Work out the finished part from the listing and answer in its coordinate system (mm). Round coordinates to 2 decimals unless told otherwise and drop trailing zeros. Write each loop counter-clockwise with the first axis right and the second up, starting at its lowest first coordinate (ties: lowest second). Pieces come first, ordered by that corner, then holes. Notation, with made-up numbers: (-39.5, 79.5) - (11.5, 79.5) arc R23 ccw to (11.5, 116.5) - close; hole circle Ø5 at (43.5, -20). An arc over 180 degrees is marked (long way). Answer as a JSON object with one key per item and string values.
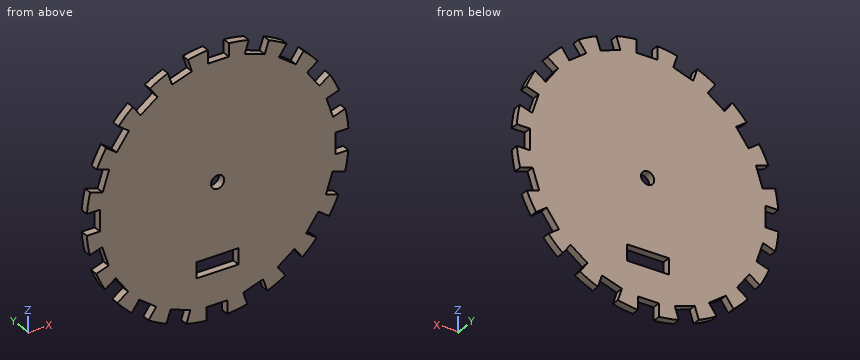
```python
from build123d import *

# Parameters (mm, degrees)
SKETCH1_R           = 50
BOSS_EXTRUDE3_DEPTH = 3
SKETCH7_R           = 2.5
CUT_EXTRUDE1_DEPTH  = 3
CUT_EXTRUDE4_START  = -3
CUT_EXTRUDE4_DEPTH  = 74.774289117
CIRPATTERN5_COUNT   = 20
SKETCH9_W           = 16
SKETCH9_H           = 6
CUT_EXTRUDE5_DEPTH  = 3


with BuildPart() as part:
    # Sketch1 → Boss-Extrude3 (new body)
    with BuildSketch(Plane(origin=(0, 0, 0), x_dir=(1, 0, 0), z_dir=(0, 1, 0))):
        with Locations(Location((0, 0, 0), (0, 0, 270))):
            Circle(SKETCH1_R)
    extrude(amount=BOSS_EXTRUDE3_DEPTH)

    # Sketch7 → Cut-Extrude1 (cut)
    with BuildSketch(Plane(origin=(0, 3, 0), x_dir=(1, 0, 0), z_dir=(0, 1, 0))):
        with Locations(Location((0, 0, 0), (0, 0, 270))):
            Circle(SKETCH7_R)
    extrude(amount=-CUT_EXTRUDE1_DEPTH, mode=Mode.SUBTRACT)

    # Sketch8 → Cut-Extrude4 (cut)
    with BuildSketch(Plane(origin=(0, 3, 0), x_dir=(1, 0, 0), z_dir=(0, 1, 0)).offset(CUT_EXTRUDE4_START)):
        Polygon((-4.300866829, 287.072728165), (-4.300866829, 49.814682018), (-4.300866829, 44.862976383), (3.699133171, 44.862976383), (3.699133171, 49.862976383), (3.699133171, 287.12102253), (0.83462867, 761.628468689), (-7.16537133, 761.580174324), align=None)
    cut_extrude4 = extrude(amount=CUT_EXTRUDE4_DEPTH, mode=Mode.SUBTRACT)

    # CirPattern5: Cut-Extrude4 ×20 about axis
    cirpattern5_axis = Axis((0, 3, 0), (0, 1, 0))
    for i in range(1, CIRPATTERN5_COUNT):
        add(cut_extrude4.rotate(cirpattern5_axis, i * 360 / CIRPATTERN5_COUNT), mode=Mode.SUBTRACT)

    # Sketch9 → Cut-Extrude5 (cut)
    with BuildSketch(Plane(origin=(0, 3, 0), x_dir=(1, 0, 0), z_dir=(0, 1, 0))):
        with Locations((-0.069626974, 30)):
            Rectangle(SKETCH9_W, SKETCH9_H)
    extrude(amount=-CUT_EXTRUDE5_DEPTH, mode=Mode.SUBTRACT)


solid = part.part
```
Item 1: A cutting plane is placed at C-C (y = 2.45). Give the number of separate pieces and of enclosed holes in the cut face, and give its area (3 significant figures).
Results found:
{"separate pieces": "1", "enclosed holes": "2", "area": "6,930 mm²"}
Item 2: A cutting plane is placed at A-A (x = 0). Write down the section's boundary in (y, z), and give its area (3 significant figures).
Results found:
{"outline": "(0, -44.86) - (3, -44.86) - (3, -33) - (0, -33) - close; (0, -27) - (3, -27) - (3, -2.5) - (0, -2.5) - close; (0, 2.5) - (3, 2.5) - (3, 44.86) - (0, 44.86) - close", "area": "236 mm²"}
Item 3: A cutting plane is placed at B-B (z = 0). Write down the section's boundary in (x, y), and give its area (3 significant figures).
Results found:
{"outline": "(-44.86, 0) - (-2.5, 0) - (-2.5, 3) - (-44.86, 3) - close; (2.5, 0) - (44.86, 0) - (44.86, 3) - (2.5, 3) - close", "area": "254 mm²"}
Item 4: Each of these flat-tipped pins is pushed along its axis until it touches: P1, Ø0.9, axis at y = 1.5, z = -47, coming from the +X side; P2, Ø0.9, axis at y = 2, z = 0, coming from the +X side; P3, Ø1.5, axis at y = 0.5, z = 36, coming from the +X side; P4, Ø4, axis at x = 0, z = 0, coming from the +Y side. Where does it stop, or does it pass through?
Results found:
{"P1": "x = 10.9", "P2": "x = 44.86", "P3": "x = 35.46", "P4": "through"}
Item 5: Consider line 1 along X through (y, z) = (2.4, 0); line 2 along Z through (x, y) = (-45, 0.8); line 3 along X through (y, z) = (0.9, 37.5). Determine where each line is inside the solid, lowest interval first.
Results found:
{"line 1": "-44.86 to -2.5, 2.5 to 44.86", "line 2": "-21.79 to -18.51, -10.1 to -3.7, 4.3 to 10.73, 19.14 to 21.79", "line 3": "-33.07 to -31.82, -24.71 to 24.71, 32.56 to 33.07"}
